Input: part model. Units: mm. Frame: model coordinates. Coordinates: 2 decimals unless noted, no trailing zeros. Order: outer loops, then holes, each group sorted by start corner. A loop starts at its lowest first (then second) coordinate and runs counter-clockwise, first axis right, second up.
from build123d import *

# Parameters (mm, degrees)
EXTRUDE_1_DEPTH     = 14
CUT_EXTRUDE_3_DEPTH = 14
SKETCH_3_R          = 6.05
EXTRUDE_2_DEPTH     = 4
CHAMFER_1_SIZE      = 0.5
SKETCH_4_R          = 1.6
CUT_EXTRUDE_4_DEPTH = 8.207143701


with BuildPart() as part:
    # Эскиз1 → Бобышка-Вытянуть1 (new body)
    with BuildSketch(Plane(origin=(0, 0, 0), x_dir=(1, 0, 0), z_dir=(0, 1, 0))):
        with BuildLine():
            Line((7, 2.5), (-7, 2.5))
            Line((-7, 2.5), (-7, -0.707143601))
            ThreePointArc((-7, -0.707143601), (0, 0), (7, -0.707143601))
            Line((7, -0.707143601), (7, 2.5))
        make_face()
    extrude(amount=EXTRUDE_1_DEPTH)

    # Эскиз2 → Вырез-Вытянуть3 (cut)
    with BuildSketch(Plane(origin=(0, 0, -2.5), x_dir=(-1, 0, 0), z_dir=(0, 0, -1))):
        with BuildLine():
            ThreePointArc((0, 0), (-4.949747468, 2.050252532), (-7, 7))
            Line((-7, 7), (-7, 0))
            Line((-7, 0), (0, 0))
        make_face()
        with BuildLine():
            Line((0, 14), (-7, 14))
            Line((-7, 14), (-7, 7))
            ThreePointArc((-7, 7), (-4.949747468, 11.949747468), (0, 14))
        make_face()
        with BuildLine():
            Line((7, 14), (0, 14))
            ThreePointArc((0, 14), (4.949747468, 11.949747468), (7, 7))
            Line((7, 7), (7, 14))
        make_face()
        with BuildLine():
            Line((7, 0), (7, 7))
            ThreePointArc((7, 7), (4.949747468, 2.050252532), (0, 0))
            Line((0, 0), (7, 0))
        make_face()
    extrude(amount=-CUT_EXTRUDE_3_DEPTH, mode=Mode.SUBTRACT)

    # Эскиз3 → Бобышка-Вытянуть2 (add)
    with BuildSketch(Plane(origin=(0, 0, -2.5), x_dir=(-1, 0, 0), z_dir=(0, 0, -1))):
        with Locations((0, 7)):
            Circle(SKETCH_3_R)
    extrude(amount=EXTRUDE_2_DEPTH)

    # Фаска1
    chamfer_1_edges = [part.edges().sort_by_distance(p)[0] for p in [
        (6.05, 7, -6.5),
    ]]
    chamfer(chamfer_1_edges, length=CHAMFER_1_SIZE)

    # Эскиз4 → Вырез-Вытянуть4 (cut, through all)
    with BuildSketch(Plane(origin=(0, 0, -6.5), x_dir=(-1, 0, 0), z_dir=(0, 0, -1))):
        with Locations((0, 7)):
            Circle(SKETCH_4_R)
    extrude(amount=-CUT_EXTRUDE_4_DEPTH, mode=Mode.SUBTRACT)


solid = part.part
Item 1: Cut plane B-B on z = -2.75. Return loops of the section in (x, y), then the cut area to 3 significant figures.
Response values:
outline: circle Ø12.1 at (0, 7); hole circle Ø3.2 at (0, 7)
area: 107 mm2
Item 2: Ray query, probe 1 along Y at (x, z) = (0, -4.25); probe 2 along Y at (x, z) = (0, -2); probe 3 along X at (y, z) = (7, -1.25). Return the intervals inside material, ascending.
Response values:
probe 1: y = 0.95 to 5.4, 8.6 to 13.05
probe 2: y = 0 to 5.4, 8.6 to 14
probe 3: x = -7 to -1.6, 1.6 to 7
Item 3: Pin query (flat end, axial travel): pin 1 Ø1 at (x, z) = (2.5, -5) entering from -Y; pin 2 Ø3 at (y, z) = (1.5, -5) entering from +X; pin 3 Ø5 at (x, y) = (1, 9) entering from +Z. Return the tip coordinate at first contact, or that it passes through.
Response values:
pin 1: stops at y = 1.29
pin 2: stops at x = 4.54
pin 3: stops at z = 0.18
Item 4: Cut plane A-A on z = -1. Return loops of the section in (x, y).
Response values:
outline: circle Ø14 at (0, 7); hole circle Ø3.2 at (0, 7)
Item 5: Draft query along X for faces 1 (the face through (1.312, 1.094, -4.226)), 2 (the face through (2, 1, -2.5)), 3 (the face through (0.35, 5.44, -3.28)), 4 (the face through (0, 5, 0)). Return one class per face: pulls with the +X half, pulls with the -X half, needs draft (parallel to the pull), parting line crosses it, or undercut.
Response values:
face 1: parting line crosses it
face 2: needs draft
face 3: undercut
face 4: undercut
